Part model, mm, in its own coordinate system. Face numbers are marked on the shaded views. Coordinates: 2 decimals unless noted, no trailing zeros. Loops run counter-clockwise (first coordinate to the right, second up) from the corner with the lowest first, then second, coordinate; pieces in that order, holes last. Notation, with made-up numbers: (69.5, 89.5) -> (76.5, 89.5) arc R38 cw to (76.5, 127.5) -> close; hole circle Ø9 at (10.25, 26.25). An arc over 180 degrees is marked (long way). One line per question, with ' | ' between items. Start each with the question number.
1) Cut at A-A (z = 15). List the corners of the cut face in (x, y).
2) Cut at C-C (y = 16). List the corners of the cut face in (x, z), plus the area to 3 significant figures.
3) Cut at D-D (x = 0). List the corners of the cut face in (y, z).
4) Drop a flat-ended pin along its axis: pin 1 (3 mm diameter, centred on x = -30, z = -15, fed in from -Y). Give the stop position or say it passes through.
5) Cut at B-B (x = -30). List the corners of the cut face in (y, z).
6) Two-plate mould, pull along X, no slides. Class the marked faces 1, 2 and 3: released by +X, released by -X, zero draft, split by the parting line, or undercut.
7) Probe L1, parallel to Z at x = 30, y = 7; L2, parallel to X at y = 25, z = 15; L3, parallel to X at y = 22, z = -15. List the from-to ranges inside material, lowest first. Write a range as from..to.
from build123d import *

# Parameters (mm, degrees)
SKETCH1_W           = 80
SKETCH1_H           = 50
SKETCH1_R           = 2.55
BOSS_EXTRUDE1_DEPTH = 32
SKETCH2_R           = 8
CUT_EXTRUDE1_DEPTH  = 50


with BuildPart() as part:
    # Sketch1 → Boss-Extrude1 (new body)
    with BuildSketch(Plane(origin=(0, 0, 0), x_dir=(1, 0, 0), z_dir=(0, 1, 0))):
        Rectangle(SKETCH1_W, SKETCH1_H)
        with Locations((-30, 15)):
            Circle(SKETCH1_R, mode=Mode.SUBTRACT)
        with Locations((30, 15)):
            Circle(SKETCH1_R, mode=Mode.SUBTRACT)
        with Locations((30, -15)):
            Circle(SKETCH1_R, mode=Mode.SUBTRACT)
        with Locations((-30, -15)):
            Circle(SKETCH1_R, mode=Mode.SUBTRACT)
    extrude(amount=BOSS_EXTRUDE1_DEPTH)

    # Sketch2 → Cut-Extrude1 (cut)
    with BuildSketch(Plane.XY.offset(25)):
        with Locations((0, 16)):
            Circle(SKETCH2_R)
    extrude(amount=-CUT_EXTRUDE1_DEPTH, mode=Mode.SUBTRACT)


solid = part.part
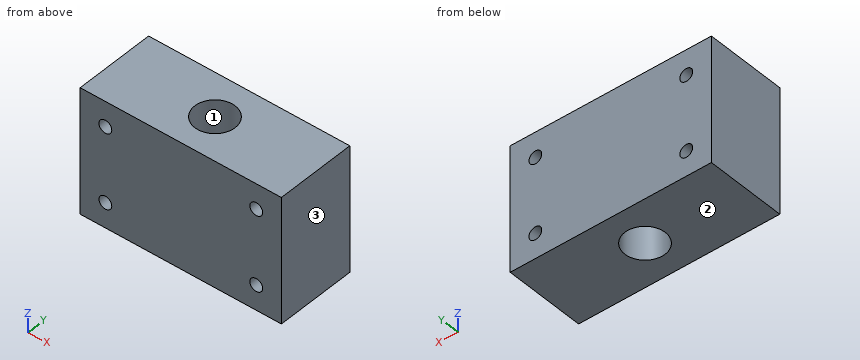
Reported:
1) outline: (-40, 0) -> (-32.55, 0) -> (-32.55, 32) -> (-40, 32) -> close; (-27.45, 0) -> (27.45, 0) -> (27.45, 32) -> (-27.45, 32) -> close; (32.55, 0) -> (40, 0) -> (40, 32) -> (32.55, 32) -> close; hole circle Ø16 at (0, 16)
2) outline: (-40, -25) -> (-8, -25) -> (-8, 25) -> (-40, 25) -> close; (8, -25) -> (40, -25) -> (40, 25) -> (8, 25) -> close; hole circle Ø5.1 at (-30, -15); hole circle Ø5.1 at (-30, 15); hole circle Ø5.1 at (30, -15); hole circle Ø5.1 at (30, 15) | area: 3,120 mm²
3) outline: (0, -25) -> (8, -25) -> (8, 25) -> (0, 25) -> close; (24, -25) -> (32, -25) -> (32, 25) -> (24, 25) -> close
4) pin 1: passes through
5) outline: (0, -25) -> (32, -25) -> (32, -17.55) -> (0, -17.55) -> close; (0, -12.45) -> (32, -12.45) -> (32, 12.45) -> (0, 12.45) -> close; (0, 17.55) -> (32, 17.55) -> (32, 25) -> (0, 25) -> close
6) face 1: undercut | face 2: zero draft | face 3: released by +X
7) L1: z = -25..-17.55, -12.45..12.45, 17.55..25 | L2: x = -40..-32.55, -27.45..27.45, 32.55..40 | L3: x = -40..-32.55, -27.45..-5.29, 5.29..27.45, 32.55..40
